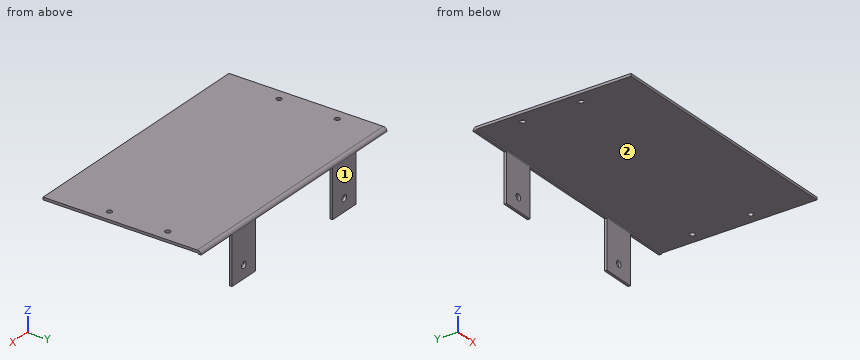
```python
from build123d import *

# Parameters (mm, degrees)
SKETCH2_W                    = 200
SKETCH2_H                    = 120
BASE_FLANGE1_DEPTH           = 2
CUT_EXTRUDE1_REACH           = 235.247
SKETCH7_R                    = 2
EDGE_FLANGE1_STRIP_W         = 9.4732
EDGE_FLANGE1_STRIP_H         = 2
EDGE_FLANGE1_STRIP_CUT_DEPTH = 200
EDGE_FLANGE1_DEPTH           = 200
CUT_EXTRUDE2_REACH           = 239.664
SKETCH11_R                   = 2.5
SKETCH11_W                   = 33.5
SKETCH11_H                   = 37.2634
SKETCH11_W_2                 = 83


# Sheet-metal steps are written as plain solids
with BuildPart() as part:
    # Sketch2 → Base-Flange1 (new body)
    with BuildSketch(Plane.XY):
        with Locations((100, 60)):
            Rectangle(SKETCH2_W, SKETCH2_H)
    extrude(amount=-BASE_FLANGE1_DEPTH)

    # Sketch7 → Cut-Extrude1 (cut, up to next)
    with BuildSketch(Plane.XY, mode=Mode.PRIVATE) as cut_extrude1_sk1:
        with Locations((8.87, 90)):
            Circle(SKETCH7_R)
    cut_extrude1_tool1 = extrude(cut_extrude1_sk1.sketch, amount=-CUT_EXTRUDE1_REACH, mode=Mode.PRIVATE) & part.part
    # Sketch7 → Cut-Extrude1 (cut, up to next)
    with BuildSketch(Plane.XY, mode=Mode.PRIVATE) as cut_extrude1_sk2:
        with Locations((8.87, 45)):
            Circle(SKETCH7_R)
    cut_extrude1_tool2 = extrude(cut_extrude1_sk2.sketch, amount=-CUT_EXTRUDE1_REACH, mode=Mode.PRIVATE) & part.part
    # Sketch7 → Cut-Extrude1 (cut, up to next)
    with BuildSketch(Plane.XY, mode=Mode.PRIVATE) as cut_extrude1_sk3:
        with Locations((191.13, 45)):
            Circle(SKETCH7_R)
    cut_extrude1_tool3 = extrude(cut_extrude1_sk3.sketch, amount=-CUT_EXTRUDE1_REACH, mode=Mode.PRIVATE) & part.part
    # Sketch7 → Cut-Extrude1 (cut, up to next)
    with BuildSketch(Plane.XY, mode=Mode.PRIVATE) as cut_extrude1_sk4:
        with Locations((191.13, 90)):
            Circle(SKETCH7_R)
    cut_extrude1_tool4 = extrude(cut_extrude1_sk4.sketch, amount=-CUT_EXTRUDE1_REACH, mode=Mode.PRIVATE) & part.part
    add(cut_extrude1_tool1.solids().sort_by_distance((8.87, 90, 0))[0], mode=Mode.SUBTRACT)
    add(cut_extrude1_tool2.solids().sort_by_distance((8.87, 45, 0))[0], mode=Mode.SUBTRACT)
    add(cut_extrude1_tool3.solids().sort_by_distance((191.13, 45, 0))[0], mode=Mode.SUBTRACT)
    add(cut_extrude1_tool4.solids().sort_by_distance((191.13, 90, 0))[0], mode=Mode.SUBTRACT)

    # Edge-Flange1 strip (across the edge) → Edge-Flange1 strip cut (cut)
    with BuildSketch(Plane(origin=(0, 120, -2), x_dir=(0, -1, 0), z_dir=(1, 0, 0))):
        with Locations((-4, -1)):
            Rectangle(EDGE_FLANGE1_STRIP_W, EDGE_FLANGE1_STRIP_H)
    extrude(amount=EDGE_FLANGE1_STRIP_CUT_DEPTH, mode=Mode.SUBTRACT)

    # Edge-Flange1 section (across the edge) → Edge-Flange1 (add)
    with BuildSketch(Plane(origin=(0, 120, -2), x_dir=(0, -1, 0), z_dir=(1, 0, 0))):
        with BuildLine():
            Line((-2, 0.7366), (-2, 38))
            Line((-2, 38), (0, 38))
            Line((0, 38), (0, 0.7366))
            ThreePointArc((0, 0.7366), (0.215745145, 0.215745145), (0.7366, 0))
            Line((0.7366, 0), (0.7366, -2))
            ThreePointArc((0.7366, -2), (-1.198468417, -1.198468417), (-2, 0.7366))
        make_face()
    extrude(amount=EDGE_FLANGE1_DEPTH)

    # Sketch11 → Cut-Extrude2 (cut, up to next)
    with BuildSketch(Plane(origin=(0, 122, 0), x_dir=(1, 0, 0), z_dir=(0, 1, 0)), mode=Mode.PRIVATE) as cut_extrude2_sk1:
        with Locations(Location((154, 30, 0), (0, 0, 270))):
            Circle(SKETCH11_R)
    cut_extrude2_tool1 = extrude(cut_extrude2_sk1.sketch, amount=-CUT_EXTRUDE2_REACH, mode=Mode.PRIVATE) & part.part
    # Sketch11 → Cut-Extrude2 (cut, up to next)
    with BuildSketch(Plane(origin=(0, 122, 0), x_dir=(1, 0, 0), z_dir=(0, 1, 0)), mode=Mode.PRIVATE) as cut_extrude2_sk2:
        with Locations(Location((46, 30, 0), (0, 0, 270))):
            Circle(SKETCH11_R)
    cut_extrude2_tool2 = extrude(cut_extrude2_sk2.sketch, amount=-CUT_EXTRUDE2_REACH, mode=Mode.PRIVATE) & part.part
    # Sketch11 → Cut-Extrude2 (cut, up to next)
    with BuildSketch(Plane(origin=(0, 122, 0), x_dir=(1, 0, 0), z_dir=(0, 1, 0)), mode=Mode.PRIVATE) as cut_extrude2_sk3:
        with Locations((183.25, 21.3683)):
            Rectangle(SKETCH11_W, SKETCH11_H)
    cut_extrude2_tool3 = extrude(cut_extrude2_sk3.sketch, amount=-CUT_EXTRUDE2_REACH, mode=Mode.PRIVATE) & part.part
    # Sketch11 → Cut-Extrude2 (cut, up to next)
    with BuildSketch(Plane(origin=(0, 122, 0), x_dir=(1, 0, 0), z_dir=(0, 1, 0)), mode=Mode.PRIVATE) as cut_extrude2_sk4:
        with Locations((100, 21.3683)):
            Rectangle(SKETCH11_W_2, SKETCH11_H)
    cut_extrude2_tool4 = extrude(cut_extrude2_sk4.sketch, amount=-CUT_EXTRUDE2_REACH, mode=Mode.PRIVATE) & part.part
    # Sketch11 → Cut-Extrude2 (cut, up to next)
    with BuildSketch(Plane(origin=(0, 122, 0), x_dir=(1, 0, 0), z_dir=(0, 1, 0)), mode=Mode.PRIVATE) as cut_extrude2_sk5:
        with Locations((16.75, 21.3683)):
            Rectangle(SKETCH11_W, SKETCH11_H)
    cut_extrude2_tool5 = extrude(cut_extrude2_sk5.sketch, amount=-CUT_EXTRUDE2_REACH, mode=Mode.PRIVATE) & part.part
    add(cut_extrude2_tool1.solids().sort_by_distance((154, 122, -30))[0], mode=Mode.SUBTRACT)
    add(cut_extrude2_tool2.solids().sort_by_distance((46, 122, -30))[0], mode=Mode.SUBTRACT)
    add(cut_extrude2_tool3.solids().sort_by_distance((183.25, 122, -21.3683))[0], mode=Mode.SUBTRACT)
    add(cut_extrude2_tool4.solids().sort_by_distance((100, 122, -21.3683))[0], mode=Mode.SUBTRACT)
    add(cut_extrude2_tool5.solids().sort_by_distance((16.75, 122, -21.3683))[0], mode=Mode.SUBTRACT)


solid = part.part
```
Source: CAD feature listing. Evaluate the final solid. Frame: model axes, mm. Face numbers are marked on the shaded views. A direction names the side the tool comes from. Round coordinates to 2 decimals unless told otherwise and drop trailing zeros. Order: outer loops, then holes, each group sorted by start corner. A loop starts at its lowest first (then second) coordinate and runs counter-clockwise, first axis right, second up. Notation, with made-up numbers: (22.5, -21) -> (48.5, -21) arc R10 ccw to (48.5, -14) -> close; hole circle Ø5 at (9, 83.25). An arc over 180 degrees is marked (long way). One line per item, written item: value. Start each with the question number.
Q1. Section query B-B (x = 154). Return the cut outline in (y, z), plus the area to 3 significant figures.
Q2. Section query C-C (y = 45). Return the cut outline in (x, z).
Q3. Access query for the marked faces 1 and 2. Directions: +Z, -Z, +X, -X, +Y, -Y. A direction counts if a zero-diameter tool reaches every point of the face in a straight line with its end or side. Return the directions, or none.
Q4. Section query A-A (z = -30). Return the cut outline in (x, y).
Q5. Pin query (flat end, axial travel): pin 1 (1 mm diameter, centred on y = 120.5, z = -18.5, fed in from +X); pin 2 (5 mm diameter, centred on x = 128.5, y = 81, fed in from -Z); pin 3 (1 mm diameter, centred on x = 95, y = 121, fed in from -Z); pin 4 (6.5 mm diameter, centred on x = 191.13, y = 45, fed in from +Z). Return the tip coordinate at first contact, or that it passes through.
Q6. Section query D-D (z = -21). Return the cut outline in (x, y).
Q7. Material intervals for probe 1 along X at (y, z) = (120.85, -30); probe 2 along Y at (x, z) = (191, -1); probe 3 along Z at (x, y) = (176.5, 80.5), sorted ascending.
Findings below:
1. outline: (0, -2) -> (119.26, -2) arc R0.74 cw to (120, -2.74) -> (120, -27.5) -> (122, -27.5) -> (122, -2.74) arc R2.74 ccw to (119.26, 0) -> (0, 0) -> close; (120, -40) -> (122, -40) -> (122, -32.5) -> (120, -32.5) -> close
1. area: 309 mm²
2. outline: (0, -2) -> (6.87, -2) -> (6.87, 0) -> (0, 0) -> close; (10.87, -2) -> (189.13, -2) -> (189.13, 0) -> (10.87, 0) -> close; (193.13, -2) -> (200, -2) -> (200, 0) -> (193.13, 0) -> close
3. face 1: +Z, -Z, +X, -X, +Y
3. face 2: -Z, +X, -X, -Y
4. outline: (33.5, 120) -> (43.5, 120) -> (43.5, 122) -> (33.5, 122) -> close; (48.5, 120) -> (58.5, 120) -> (58.5, 122) -> (48.5, 122) -> close; (141.5, 120) -> (151.5, 120) -> (151.5, 122) -> (141.5, 122) -> close; (156.5, 120) -> (166.5, 120) -> (166.5, 122) -> (156.5, 122) -> close
5. pin 1: x = 166.5
5. pin 2: z = -2
5. pin 3: z = -2.74
5. pin 4: z = 0
6. outline: (33.5, 120) -> (58.5, 120) -> (58.5, 122) -> (33.5, 122) -> close; (141.5, 120) -> (166.5, 120) -> (166.5, 122) -> (141.5, 122) -> close
7. probe 1: 33.5 to 43.5, 48.5 to 58.5, 141.5 to 151.5, 156.5 to 166.5
7. probe 2: 0 to 43, 47 to 88, 92 to 121.38
7. probe 3: -2 to 0
